Geometry check sheet. Reference: drawing and pictorial views, mm from the part's lowest x, y, z. A direction names the side the tool comes from. Round coordinates to 2 decimals unless told otherwise and drop trailing zeros. Write each loop counter-clockwise with the first axis right and the second up, starting at its lowest first coordinate (ties: lowest second). Pieces come first, ordered by that corner, then holes. Notation, with made-up numbers: M 83.5,89 L 107.5,89 A18 ccw 107.5,122 Z; hole C -29.5,51 d5. An arc over 180 degrees is marked long. Answer in a Markdown table with one row per item. Add a question column.
1. Sectioned sample at B-B on y = 15. Record the cut outline in (x, z), plus the area to 3 significant figures.
2. Material ranges on probe 1 along Z at (x, y) = (13.25, 8); probe 2 along Y at (x, z) = (13, 3.25); probe 3 along X at (y, z) = (16.5, 22.75), recorded low to high.
3. Go/stop test with flat-tipped pins: pin 1 Ø2 at (x, y) = (11.5, 9.5) entering from -Z; pin 2 Ø3 at (y, z) = (14, 18.5) entering from +X; pin 3 Ø1 at (y, z) = (20.5, 22.5) entering from +X. Record where each tip stops, or that it passes through.
4. Set-up check for the marked faces 1 and 2: record each of +Z, -Z, +X, -X, +Y, -Y from which the full face is reachable in a straight line by a thin tool's end or side.
5. Draft check along Z on the marked faces 3 and 4. Enter one of: pulls with the +Z half, pulls with the -Z half, needs draft (parallel to the pull), parting line crosses it, or undercut.
6. Sectioned sample at A-A on x = 13.5. Record the cut outline in (y, z), plus the area to 3 significant figures.
7. Sectioned sample at C-C on y = 23.75. Record the cut outline in (x, z).
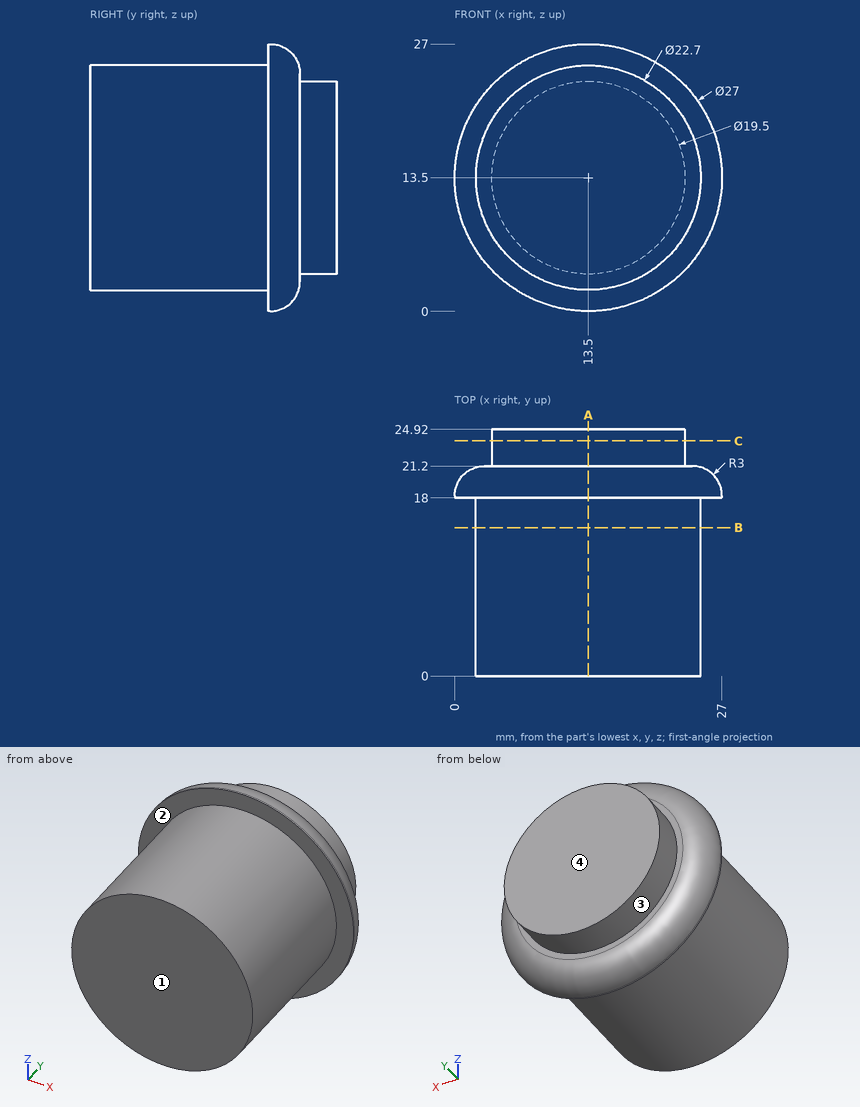
Geometry check:
| question | item | result |
|---|---|---|
| 1 | outline | C 13.5,13.5 d22.7 |
| 1 | area | 405 mm2 |
| 2 | probe 1 | z = 2.15 to 24.85 |
| 2 | probe 2 | y = 0 to 21.2 |
| 2 | probe 3 | x = 6.92 to 20.08 |
| 3 | pin 1 | stops at z = 2.19 |
| 3 | pin 2 | stops at x = 24.3 |
| 3 | pin 3 | stops at x = 22.92 |
| 4 | face 1 | +Z, -Z, +X, -X, -Y |
| 4 | face 2 | -Y |
| 5 | face 3 | parting line crosses it |
| 5 | face 4 | needs draft |
| 6 | outline | M 0,2.15 L 18,2.15 L 18,0 L 18.2,0 A3 ccw 21.2,3 L 21.2,3.75 L 24.92,3.75 L 24.92,23.25 L 21.2,23.25 L 21.2,24 A3 ccw 18.2,27 L 18,27 L 18,24.85 L 0,24.85 Z |
| 6 | area | 564 mm2 |
| 7 | outline | C 13.5,13.5 d19.5 |
